The listing builds one solid part. Answer for the finished solid, in the listing's coordinates (mm). A direction names the side the tool comes from. Give positions to 0.01 mm unless a question says otherwise; leave off trailing zeros. Use a Markdown table: item, result. Add a question column.
1) For faces 1 (the face through (4, 0, 184)), 2 (the face through (4, 32, 1.8)), determine the directions among +Z, -Z, +X, -X, +Y, -Y from which every point of the face is accessible in a straight line to the end or side of a thin tool.
2) A flat-ended cylindrical pin translates along its axis: pin 1 (1.5 mm diameter, centred on x = 42.5, y = 21.5, fed in from +Z). Find the tip coordinate at first contact, or state that the pin passes through.
3) Straight lines are drawn through the part: line 1 (Y direction, x = -124, z = 237); line 2 (Z direction, x = -57, y = 4). For each, find the intervals that lie inside material, in ascending order.
from build123d import *

# Parameters (mm, degrees)
F2_DEPTH = 261
F3_R     = 3.6
F4_R     = 0.89999


# Not quite as in the source:
# - a fillet or chamfer is up to 0.001 mm smaller than in the source, because OpenCascade refuses the exact size


with BuildPart() as f2:
    # F1 (on Right) → F2 (new body)
    with BuildSketch(Plane.YZ):
        Polygon((0, 360), (0, 0), (59.5, 0), (59.5, 1.8), (1.8, 1.8), (1.8, 360), align=None)
    extrude(amount=F2_DEPTH)

    # F3
    f3_edges = [f2.edges().sort_by_distance(p)[0] for p in [
        (130.5, 1.8, 1.8),
        (130.5, 0, 0),
    ]]
    fillet(f3_edges, radius=F3_R)

    # F4 (radius 0.9 in the source; OpenCascade refuses exactly that, so slightly less here)
    f4_edges = [f2.edges().sort_by_distance(p)[0] for p in [
        (261, 32.45, 1.8),
        (261, 31.55, 0),
        (130.5, 59.5, 1.8),
        (130.5, 59.5, 0),
        (261, 1.8, 182.7),
        (261, 0, 181.8),
        (130.5, 0, 360),
        (130.5, 1.8, 360),
        (261, 1.054416, 1.054416),
    ]]
    fillet(f4_edges, radius=F4_R)

    # F5: F2 across face


with BuildPart() as f2_1:
    add(f2.part)
    add(f2.part.mirror(Plane(origin=(0, 4.9930290886, 155.2430290886), x_dir=(0, 1, 0), z_dir=(-1, 0, 0))))


solid = f2_1.part
The answers:
| question | item | result |
|---|---|---|
| 1 | face 1 | +Z, -Z, +X, -X, -Y |
| 1 | face 2 | +Z, +X, -X, +Y |
| 2 | pin 1 | z = 1.8 |
| 3 | line 1 | 0 to 1.8 |
| 3 | line 2 | 0 to 2.08 |
